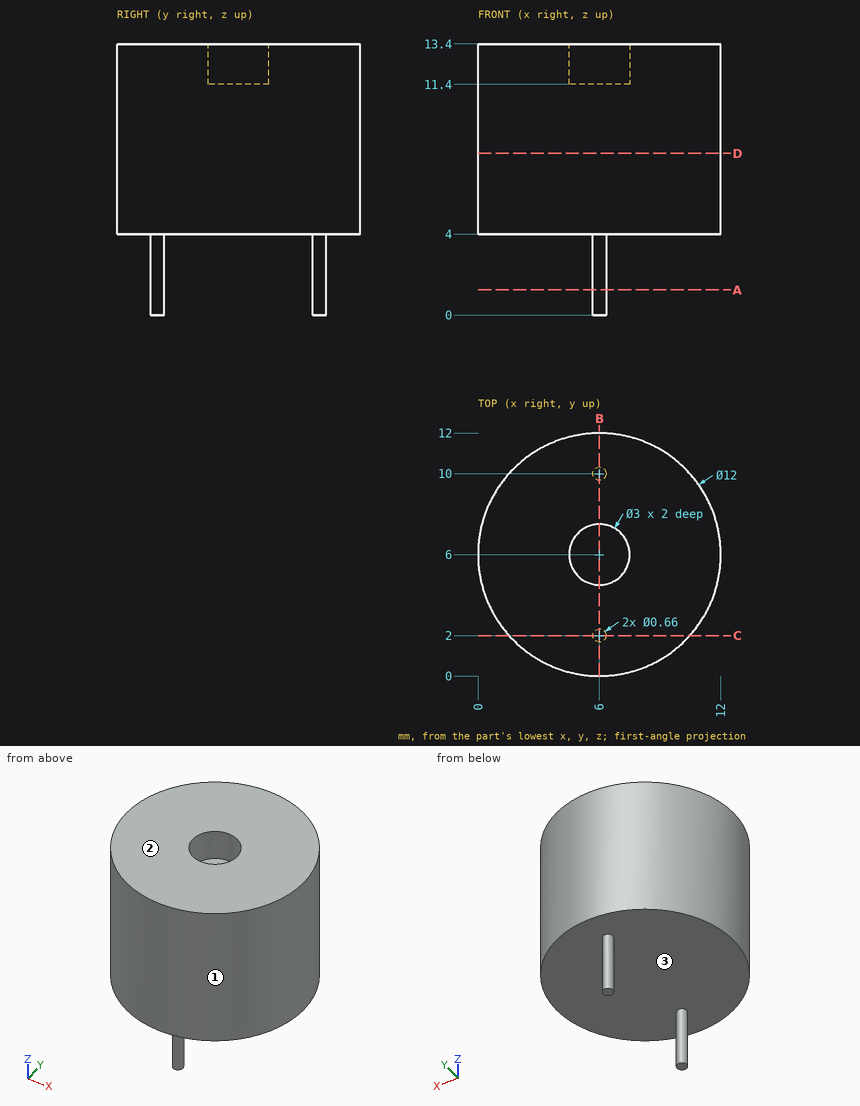
Here's the drawing with two shaded views (mm, measured from the low corner). I have some questions. Give positions to 0.01 mm unless a question says otherwise; leave off trailing zeros. Write each loop counter-clockwise with the first axis right and the second up, starting at its lowest first coordinate (ties: lowest second). Pieces come first, ordered by that corner, then holes. Notation, with made-up numbers: (62.5, 34.25) -> (97.5, 34.25) arc R15 ccw to (97.5, 43.25) -> close; hole circle Ø3 at (-22.75, -3.75). An arc over 180 degrees is marked (long way). Answer as a JSON object with one key per item and string values. Group by question number.
Item 1: We'd pull the mould along Z, two halves only. Please class the marked faces 1, 2 and 3: +Z half, -Z half, draft (parallel to the pull), parting line (faces both ways), or undercut.
Item 2: I'm going to push flat-ended pins straight in: P1, Ø5, axis at x = 6, y = 6, coming from the +Z side; P2, Ø5, axis at y = 1.5, z = 4, coming from the +X side; P3, Ø3, axis at x = 10.5, z = 12, coming from the +Y side; P4, Ø4, axis at x = 6, y = 5, coming from the -Z side. Where does each tip first touch, or does it pass through?
Item 3: Please list where these lines run through material, in increasing order: line 1 (Y direction, x = 6, z = 12.2); line 2 (Z direction, x = 4.75, y = 0.5); line 3 (X direction, y = 2, z = 2). Write a range as [from, to].
Item 4: Suppose I cut it at B-B (x = 6). Please give me the cut outline in (y, z).
Item 5: Suppose I cut it at C-C (y = 2). Please give me the cut outline in (x, z), plus the area to 3 significant figures.
Item 6: Suppose I cut it at A-A (z = 1.25). Please give me the cut outline in (x, y).
Item 7: Suppose I cut it at D-D (z = 8). Please give me the cut outline in (x, y).
Findings:
{
 "1": {"face 1": "draft", "face 2": "+Z half", "face 3": "-Z half"},
 "2": {"P1": "stops at z = 13.4", "P2": "stops at x = 11.66", "P3": "stops at y = 11.2", "P4": "stops at z = 4"},
 "3": {"line 1": "y = [0, 4.5], [7.5, 12]", "line 2": "z = [4, 13.4]", "line 3": "x = [5.67, 6.33]"},
 "4": {"outline": "(0, 4) -> (1.67, 4) -> (1.67, 0) -> (2.33, 0) -> (2.33, 4) -> (9.67, 4) -> (9.67, 0) -> (10.33, 0) -> (10.33, 4) -> (12, 4) -> (12, 13.4) -> (7.5, 13.4) -> (7.5, 11.4) -> (4.5, 11.4) -> (4.5, 13.4) -> (0, 13.4) -> close"},
 "5": {"outline": "(1.53, 4) -> (5.67, 4) -> (5.67, 0) -> (6.33, 0) -> (6.33, 4) -> (10.47, 4) -> (10.47, 13.4) -> (1.53, 13.4) -> close", "area": "86.7 mm²"},
 "6": {"outline": "circle Ø0.66 at (6, 2); circle Ø0.66 at (6, 10)"},
 "7": {"outline": "circle Ø12 at (6, 6)"}
}
